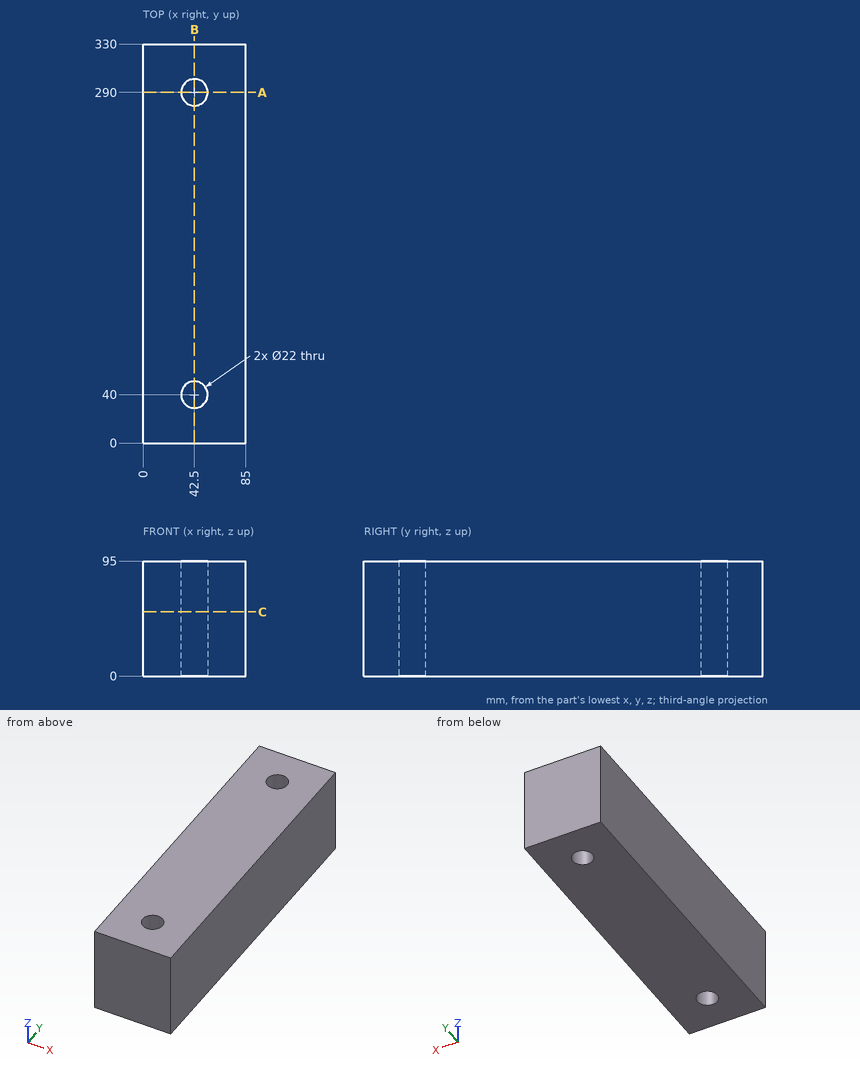
Part print with two shaded views. Sizes in mm from the minimum x, y, z corner. Give positions to 0.01 mm unless a question says otherwise; leave off trailing zeros. Order: outer loops, then holes, each group sorted by start corner. A loop starts at its lowest first (then second) coordinate and runs counter-clockwise, first axis right, second up.
(1) Flat gauge pins, fed straight in: pin 1 (10 mm diameter, centred on y = 291.5, z = 11, fed in from -X); pin 2 (17.5 mm diameter, centred on x = 42.5, y = 40, fed in from -Z). Where does each tip first touch, or does it go through?
(2) Saw through at B-B, the plane x = 42.5. Give the cut face in (y, z), then the cut area to 3 significant figures.
(3) Drill centre lines: L1, parallel to Y at x = 42, z = 45; L2, parallel to X at y = 40, z = 22; L3, parallel to Y at x = 35, z = 55. Where is each one in solid material? Low to high.
(4) Saw through at C-C, the plane z = 53. Give the cut face in (x, y).
(5) Saw through at A-A, the plane y = 290. Give the cut face in (x, z), then the cut area to 4 significant figures.
Results found:
1. pin 1: stops at x = 0
1. pin 2: passes through
2. outline: (0, 0) - (29, 0) - (29, 95) - (0, 95) - close; (51, 0) - (279, 0) - (279, 95) - (51, 95) - close; (301, 0) - (330, 0) - (330, 95) - (301, 95) - close
2. area: 27,200 mm2
3. L1: y = 0 to 29.01, 50.99 to 279.01, 300.99 to 330
3. L2: x = 0 to 31.5, 53.5 to 85
3. L3: y = 0 to 31.95, 48.05 to 281.95, 298.05 to 330
4. outline: (0, 0) - (85, 0) - (85, 330) - (0, 330) - close; hole circle Ø22 at (42.5, 40); hole circle Ø22 at (42.5, 290)
5. outline: (0, 0) - (31.5, 0) - (31.5, 95) - (0, 95) - close; (53.5, 0) - (85, 0) - (85, 95) - (53.5, 95) - close
5. area: 5,985 mm2
